For this review, use the dimensioned drawing (mm, ordinates from the lowest corner) and the shaded views. A direction names the side the tool comes from. Give positions to 0.01 mm unless a question says otherwise; leave off trailing zeros. Order: outer loops, then holes, each group sorted by start corner. A loop starts at its lowest first (then second) coordinate and runs counter-clockwise, first axis right, second up. Notation, with made-up numbers: M 89.5,44.5 L 135.5,44.5 A23 cw 135.5,58.5 Z; hole C 83,84.25 d10. An arc over 180 degrees is marked long. Use CSV: the item, a comma, the result in double quotes. Start each with the question number.
(1) Consider section D-D (x = 21.5). Write out the cut boundary in (y, z) (1 decimal).
(2) Tool access review of the marked faces 1 and 2: name each direction out of +Z, -Z, +X, -X, +Y, -Y from which nothing blocks a thin tool from reaching the whole face with its end or side.
(3) Clearance check with flat-ended pins moving along their axes: P1, Ø12, axis at x = 11.5, z = 19.5, coming from the -Y side; P2, Ø13, axis at x = 12, y = 23.5, coming from the -Z side. State where each tip first meets the part, or that it passes through.
(4) Consider section C-C (y = 17). Write out the cut boundary in (x, z).
(5) Consider section A-A (x = 14.25). Write out the cut boundary in (y, z).
(6) Consider section B-B (z = 15.5). Write out the cut boundary in (x, y).
(7) Wall thickness on L1, parallel to X at y = 31.85, z = 13; L2, parallel to Z at x = 6, y = 17; L3, parallel to Y at x = 21, z = 31.95 (1 decimal): over which ranges is each line inside the solid? List them lowest first. Write a range as from..to.
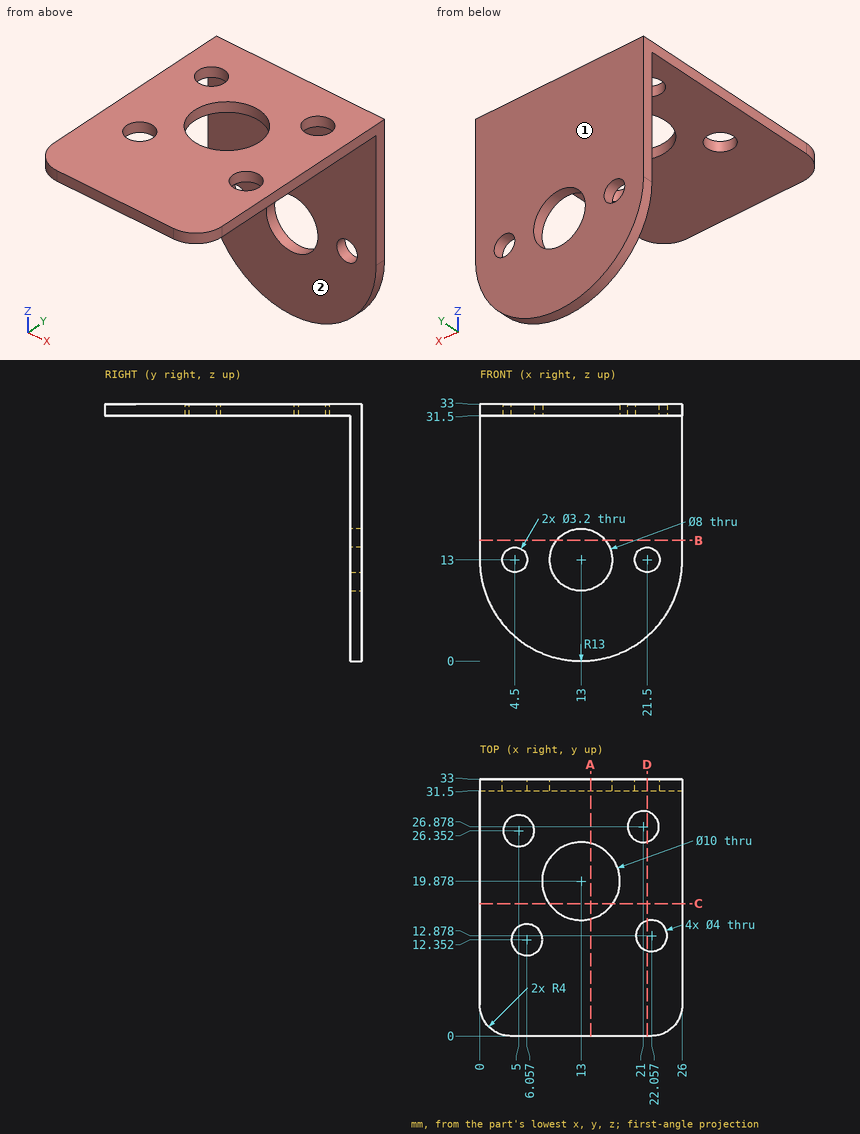
Check result:
1,outline,"M 0,31.5 L 11,31.5 L 11,33 L 0,33 Z; M 14.8,31.5 L 24.9,31.5 L 24.9,33 L 14.8,33 Z; M 28.8,31.5 L 31.5,31.5 L 31.5,14.6 L 33,14.6 L 33,33 L 28.8,33 Z; M 31.5,3.2 L 33,3.2 L 33,11.4 L 31.5,11.4 Z"
2,face 1,"+Z, -Z, +X, -X, +Y"
2,face 2,"-Z, +X, -X, -Y"
3,P1,"stops at y = 31.5"
3,P2,"stops at z = 31.5"
4,outline,"M 0,31.5 L 8.91,31.5 L 8.91,33 L 0,33 Z; M 17.09,31.5 L 26,31.5 L 26,33 L 17.09,33 Z"
5,outline,"M 0,31.5 L 15.04,31.5 L 15.04,33 L 0,33 Z; M 24.72,31.5 L 31.5,31.5 L 31.5,16.8 L 33,16.8 L 33,33 L 24.72,33 Z; M 31.5,0.06 L 33,0.06 L 33,9.2 L 31.5,9.2 Z"
6,outline,"M 0,31.5 L 9.88,31.5 L 9.88,33 L 0,33 Z; M 16.12,31.5 L 26,31.5 L 26,33 L 16.12,33 Z"
7,L1,"x = 0..2.9, 6.1..9, 17..19.9, 23.1..26"
7,L2,"z = 31.5..33"
7,L3,"y = 0..11.2, 14.6..24.9, 28.9..33"
